from build123d import *

# Parameters (mm, degrees)
SKETCH2_W            = 22.657552765
SKETCH2_H            = 51.264295363
BOSS_EXTRUDE1_DEPTH  = 2
SKETCH3_W            = 22.657552765
SKETCH3_H            = 51.264295363
SKETCH3_W_2          = 20.905191144
SKETCH3_H_2          = 49.290834071
BOSS_EXTRUDE2_DEPTH  = 21
BOSS_EXTRUDE3_DEPTH  = 78
SKETCH6_W            = 21.285297843
SKETCH6_H            = 14.278933142
CUT_EXTRUDE1_DEPTH   = 80
SKETCH11_R           = 14
BOSS_EXTRUDE4_DEPTH  = 50
BOSS_EXTRUDE4_DRAFT  = -30
SKETCH12_R           = 36.30995568
CUT_EXTRUDE2_DEPTH   = 51
CUT_EXTRUDE2_DRAFT   = -30
SKETCH14_R           = 5
CUT_EXTRUDE4_DEPTH   = 22
SKETCH15_W           = 15.409943134
SKETCH15_H           = 1.668824362
CUT_EXTRUDE5_DEPTH   = 22
SKETCH16_W           = 111.818738814
SKETCH16_H           = 164.067511329
BOSS_EXTRUDE10_DEPTH = 6
BOSS_EXTRUDE11_DEPTH = 14
CUT_EXTRUDE6_DEPTH   = 14


with BuildPart() as part:
    # Sketch2 → Boss-Extrude1 (new body)
    with BuildSketch(Plane(origin=(0, 0, 0), x_dir=(1, 0, 0), z_dir=(0, 1, 0))):
        with Locations((11.328776383, 25.632147682)):
            Rectangle(SKETCH2_W, SKETCH2_H)
    extrude(amount=BOSS_EXTRUDE1_DEPTH)

    # Sketch3 → Boss-Extrude2 (add)
    with BuildSketch(Plane(origin=(0, 2, 0), x_dir=(1, 0, 0), z_dir=(0, 1, 0))):
        with Locations((11.328776383, 25.632147682)):
            Rectangle(SKETCH3_W, SKETCH3_H)
        with Locations((11.328776383, 25.598752808)):
            Rectangle(SKETCH3_W_2, SKETCH3_H_2, mode=Mode.SUBTRACT)
    extrude(amount=BOSS_EXTRUDE2_DEPTH)

    # Sketch5 → Boss-Extrude3 (add)
    with BuildSketch(Plane(origin=(0, 23, 0), x_dir=(1, 0, 0), z_dir=(0, 1, 0))):
        Polygon((22.657552765, 37.450286435), (22.657552765, 51.264295363), (0, 51.264295363), (0, 35.580664168), (22.657552765, 35.580664168), align=None)
    extrude(amount=BOSS_EXTRUDE3_DEPTH)

    # Sketch6 → Cut-Extrude1 (cut)
    with BuildSketch(Plane(origin=(0, 101, 0), x_dir=(1, 0, 0), z_dir=(0, 1, 0))):
        with Locations((11.316093437, 43.486003654)):
            Rectangle(SKETCH6_W, SKETCH6_H)
    extrude(amount=-CUT_EXTRUDE1_DEPTH, mode=Mode.SUBTRACT)


with BuildPart() as boss_extrude4_tool:
    # Sketch11 → Boss-Extrude4 (with draft: the straight prism first)
    with BuildSketch(Plane(origin=(0, 101, 0), x_dir=(1, 0, 0), z_dir=(0, 1, 0))):
        with Locations((11.328776383, 43.422479766)):
            Circle(SKETCH11_R)
    extrude(amount=BOSS_EXTRUDE4_DEPTH)
    # Boss-Extrude4: the draft: its side faces are tilted about the plane it starts from
    boss_extrude4_sides = [boss_extrude4_tool.faces().sort_by_distance(p)[0] for p in [
        (-2.671223617, 126, -43.422479766),
    ]]
    draft(boss_extrude4_sides, Plane(origin=(0, 101, 0), x_dir=(1, 0, 0), z_dir=(0, 1, 0)), BOSS_EXTRUDE4_DRAFT)


with BuildPart() as part_1:
    add(part.part)

    # Boss-Extrude4: add boss_extrude4_tool
    add(boss_extrude4_tool.part)


with BuildPart() as cut_extrude2_tool:
    # Sketch12 → Cut-Extrude2 (with draft: the straight prism first)
    with BuildSketch(Plane(origin=(0, 151, 0), x_dir=(1, 0, 0), z_dir=(0, 1, 0))):
        with Locations((11.328776383, 43.422479766)):
            Circle(SKETCH12_R)
    extrude(amount=-CUT_EXTRUDE2_DEPTH)
    # Cut-Extrude2: the draft: its side faces are tilted about the plane it starts from
    cut_extrude2_sides = [cut_extrude2_tool.faces().sort_by_distance(p)[0] for p in [
        (-24.981179297, 125.5, -43.422479766),
    ]]
    draft(cut_extrude2_sides, Plane(origin=(0, 151, 0), x_dir=(1, 0, 0), z_dir=(0, 1, 0)), CUT_EXTRUDE2_DRAFT)


with BuildPart() as part_2:
    add(part_1.part)

    # Cut-Extrude2: cut by cut_extrude2_tool
    add(cut_extrude2_tool.part, mode=Mode.SUBTRACT)

    # Sketch14 → Cut-Extrude4 (cut)
    with BuildSketch(Plane.XY):
        with Locations((11.657552765, 11.076385635)):
            Circle(SKETCH14_R)
    extrude(amount=-CUT_EXTRUDE4_DEPTH, mode=Mode.SUBTRACT)

    # Sketch15 → Cut-Extrude5 (cut)
    with BuildSketch(Plane.XY):
        with Locations((10.856611193, 18.879859243)):
            Rectangle(SKETCH15_W, SKETCH15_H)
    extrude(amount=-CUT_EXTRUDE5_DEPTH, mode=Mode.SUBTRACT)

    # Sketch16 → Boss-Extrude10 (add)
    with BuildSketch(Plane.XZ):
        with Locations((11.63043448, -23.117453155)):
            Rectangle(SKETCH16_W, SKETCH16_H)
    extrude(amount=BOSS_EXTRUDE10_DEPTH)

    # Sketch17 → Boss-Extrude11 (add)
    with BuildSketch(Plane(origin=(0, 0, 0), x_dir=(1, 0, 0), z_dir=(0, 1, 0))):
        Polygon((-44.278934927, -19.158930428), (-22.558261241, -19.158930428), (-22.558261241, -58.91630251), (-18.859616668, -58.91630251), (-18.859616668, -15.83203433), (-44.278934927, -15.83203433), align=None)
    extrude(amount=BOSS_EXTRUDE11_DEPTH)

    # Sketch18 → Cut-Extrude6 (cut)
    with BuildSketch(Plane(origin=(0, 2, 0), x_dir=(1, 0, 0), z_dir=(0, 1, 0))):
        Polygon((4.238517858, 49.520767008), (19.451065942, 49.052935497), (19.451065942, 47.510847256), (4.238517858, 47.978678766), align=None)
    extrude(amount=-CUT_EXTRUDE6_DEPTH, mode=Mode.SUBTRACT)


solid = part_2.part
Geometry check sheet. Reference: the model listing, model coordinates, mm. A direction names the side the tool comes from. Coordinates: 2 decimals unless noted, no trailing zeros. Loops run counter-clockwise (first coordinate to the right, second up) from the corner with the lowest first, then second, coordinate; pieces in that order, holes last. Notation, with made-up numbers: (-29, -10.75) - (-20, -10.75) arc R33 ccw to (-20, 18.25) - close; hole circle Ø7 at (66, 13). An arc over 180 degrees is marked (long way). Use one line per item in the form item = value. Start each with the question number.
Item 1: Section check C-C, the plane y = 122. Enter the section's corners in (x, z).
Item 2: Mould release check, pull along Z, two halves, no side actions. Record for faces 1 (the face through (0.4, 23, -12.6)), 2 (the face through (-31, 7, 15.832)), 3 (the face through (11, 2, -26)): +Z half, -Z half, draft (parallel to the pull), parting line (faces both ways), or undercut.
Item 3: Thickness scan on probe 1 along Z at (x, y) = (4, 64); probe 2 along X at (y, z) = (11, -25.5); probe 3 along X at (y, z) = (131, -22). Record the ranges inside material, lowest first.
Item 4: Section check D-D, the plane z = 6.5. Enter the section's corners in (x, y), and give its area (3 significant figures).
Item 5: Tool access check on faces 4 (the face through (22.658, 39, -37)), 5 (the face through (-18.86, 7, 38)), 6 (the face through (0, 39, -37)), 7 (the face through (-22.558, 7, 39)), 8 (the face through (19, 101, -44)). Record the directions out of +Z, -Z, +X, -X, +Y, -Y that give a thin tool (end or side, any length) a straight path to the whole face; none if there is none.
Item 6: Section check A-A, the plane y = 64. Enter the section's corners in (x, z), and give its area (3 significant figures).
Item 7: Section check B-B, the plane z = 28. Enter the section's corners in (x, y).
Item 8: Gauge pin test, flat ends, axial feed: pin 1 (1 mm diameter, centred on y = 19, z = -0.5, fed in from -X); pin 2 (17.5 mm diameter, centred on x = -32.5, z = 35.5, fed in from +Y); pin 3 (16.5 mm diameter, centred on x = 9.5, z = -25.5, fed in from +Y). Record the tip position at first contact, or that the pin passes through.
Computed:
q1.outline = circle Ø52.25 at (11.33, -43.42); hole circle Ø39.13 at (11.33, -43.42)
q2.face_1 = draft
q2.face_2 = -Z half
q2.face_3 = undercut
q3.probe_1 = -51.26 to -50.63, -36.35 to -35.58
q3.probe_2 = 0 to 0.88, 21.78 to 22.66
q3.probe_3 = -11.52 to -1.09, 23.75 to 34.18
q4.outline = (-44.28, -6) - (67.54, -6) - (67.54, 0) - (-44.28, 0) - close
q4.area = 671 mm2
q5.face_4 = +Z, -Z, +X
q5.face_5 = +Z, -Z, +X, +Y
q5.face_6 = +Z, -Z, -X
q5.face_7 = +Z, -X, +Y
q5.face_8 = none
q6.outline = (0, -51.26) - (22.66, -51.26) - (22.66, -35.58) - (0, -35.58) - close; hole (0.67, -50.63) - (21.96, -50.63) - (21.96, -36.35) - (0.67, -36.35) - close
q6.area = 51.4 mm2
q7.outline = (-44.28, -6) - (67.54, -6) - (67.54, 0) - (-18.86, 0) - (-18.86, 14) - (-22.56, 14) - (-22.56, 0) - (-44.28, 0) - close
q8.pin_1 = 0
q8.pin_2 = 0
q8.pin_3 = 133.6
